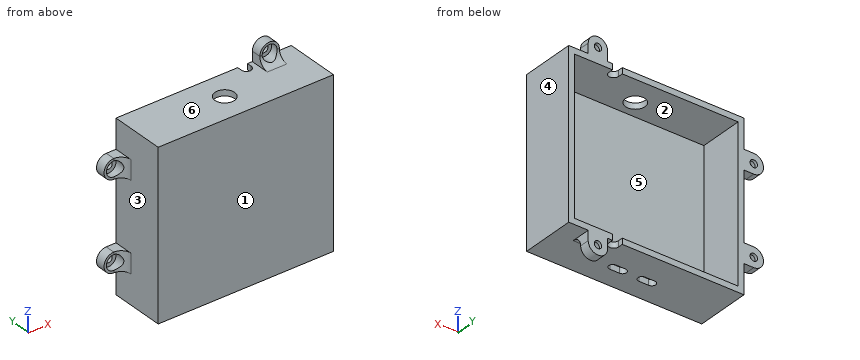
from build123d import *

# Parameters (mm, degrees)
SKETCH1_W                                      = 90
SKETCH1_H                                      = 85
BOSS_EXTRUDE1_DEPTH                            = 28
SHELL1_T                                       = -3
SHELL1_THICKNESS_2_FACE_W                      = 79
SHELL1_THICKNESS_2_FACE_H                      = 84
SHELL1_THICKNESS_2_DEPTH                       = 2.25
CUT_EXTRUDE1_REACH                             = 102.17
SKETCH2_R                                      = 5.05
BOSS_EXTRUDE2_DEPTH                            = 5
BOSS_EXTRUDE3_DEPTH                            = 5
CBORE_FOR_6_SOCKET_HEAD_CAP_SCREW1_D           = 3.7973
CBORE_FOR_6_SOCKET_HEAD_CAP_SCREW1_CBORE_D     = 7.62
CBORE_FOR_6_SOCKET_HEAD_CAP_SCREW1_CBORE_DEPTH = 3.5052
FILLET1_R                                      = 5
CUT_EXTRUDE2_DEPTH                             = 114.287245531
CUT_EXTRUDE4_REACH                             = 124.741


with BuildPart() as part:
    # Sketch1 → Boss-Extrude1 (new body)
    with BuildSketch(Plane(origin=(0, 0, 0), x_dir=(1, 0, 0), z_dir=(0, 1, 0))):
        Rectangle(SKETCH1_W, SKETCH1_H)
    extrude(amount=BOSS_EXTRUDE1_DEPTH)

    # Shell1
    shell1_openings = [part.faces().sort_by_distance(p)[0] for p in [
        (0, 28, 0),
    ]]
    offset(amount=SHELL1_T, openings=shell1_openings, kind=Kind.INTERSECTION)

    # Shell1 thickness 2 face (on inner face of the shell) → Shell1 thickness 2 (add)
    with BuildSketch(Plane(origin=(0, 3, 0), x_dir=(0, 0, -1), z_dir=(0, -1, 0))):
        Rectangle(SHELL1_THICKNESS_2_FACE_W, SHELL1_THICKNESS_2_FACE_H)
    extrude(amount=-SHELL1_THICKNESS_2_DEPTH)

    # Sketch2 → Cut-Extrude1 (cut, up to next)
    with BuildSketch(Plane.XY.offset(42.5), mode=Mode.PRIVATE) as cut_extrude1_sk1:
        with Locations((0, 14)):
            Circle(SKETCH2_R)
    cut_extrude1_tool1 = extrude(cut_extrude1_sk1.sketch, amount=-CUT_EXTRUDE1_REACH, mode=Mode.PRIVATE) & part.part
    add(cut_extrude1_tool1.solids().sort_by_distance((0, 14, 42.5))[0], mode=Mode.SUBTRACT)

    # Sketch3 → Boss-Extrude2 (add)
    with BuildSketch(Plane(origin=(0, 28, 0), x_dir=(1, 0, 0), z_dir=(0, 1, 0))):
        with BuildLine():
            Line((-50, 27.5), (-45, 27.5))
            Line((-45, 27.5), (-45, 17.5))
            Line((-45, 17.5), (-50, 17.5))
            ThreePointArc((-50, 17.5), (-55, 22.5), (-50, 27.5))
        make_face()
    boss_extrude2 = extrude(amount=-BOSS_EXTRUDE2_DEPTH)

    # Mirror1: Boss-Extrude2 across plane
    add(boss_extrude2.mirror(Plane.XY))

    # Sketch4 → Boss-Extrude3 (add)
    with BuildSketch(Plane(origin=(0, 28, 0), x_dir=(1, 0, 0), z_dir=(0, 1, 0))):
        with BuildLine():
            Line((25, 47.5), (25, 42.5))
            Line((25, 42.5), (35, 42.5))
            Line((35, 42.5), (35, 47.5))
            ThreePointArc((35, 47.5), (30, 52.5), (25, 47.5))
        make_face()
    boss_extrude3 = extrude(amount=-BOSS_EXTRUDE3_DEPTH)

    # Mirror2: Boss-Extrude3 across plane
    add(boss_extrude3.mirror(Plane.XY))

    # CBORE for #6 Socket Head Cap Screw1 (through all)
    with Locations(Plane(origin=(0, 23, 0), x_dir=(-1, 0, 0), z_dir=(0, -1, 0))):
        with Locations((-30, 47.5), (-30, -47.5), (50, -22.5), (50, 22.5)):
            CounterBoreHole(CBORE_FOR_6_SOCKET_HEAD_CAP_SCREW1_D / 2, CBORE_FOR_6_SOCKET_HEAD_CAP_SCREW1_CBORE_D / 2, CBORE_FOR_6_SOCKET_HEAD_CAP_SCREW1_CBORE_DEPTH)

    # Fillet1
    # the kernel refuses this fillet: 5 mm, written as the material it adds along each edge
    with BuildSketch(Plane(origin=(25, 23, -42.5), x_dir=(0, -1, 0), z_dir=(1, 0, 0))) as fillet1_piece_1_section:
        with BuildLine():
            CenterArc((FILLET1_R, FILLET1_R), FILLET1_R, 180, 90)
            Line((0, FILLET1_R), (0, 0))
            Line((0, 0), (FILLET1_R, 0))
        make_face()
    fillet1_piece_1 = extrude(amount=10, mode=Mode.PRIVATE)
    fillet1_piece_1 = fillet1_piece_1 - Plane(origin=(30, 21.803509944, -47.5), x_dir=(-1, 0, 0), z_dir=(0, -1, 0)) * Cylinder(3.81, 40, mode=Mode.PRIVATE)
    add(fillet1_piece_1)
    with BuildSketch(Plane(origin=(25, 23, 42.5), x_dir=(0, -1, 0), z_dir=(1, 0, 0))) as fillet1_piece_2_section:
        with BuildLine():
            CenterArc((FILLET1_R, -FILLET1_R), FILLET1_R, 90, 90)
            Line((0, -FILLET1_R), (0, 0))
            Line((0, 0), (FILLET1_R, 0))
        make_face()
    fillet1_piece_2 = extrude(amount=10, mode=Mode.PRIVATE)
    fillet1_piece_2 = fillet1_piece_2 - Plane(origin=(30, 21.803509344, 47.5), x_dir=(-1, 0, 0), z_dir=(0, -1, 0)) * Cylinder(3.81, 40, mode=Mode.PRIVATE)
    add(fillet1_piece_2)
    with BuildSketch(Plane(origin=(-45, 23, -27.5), x_dir=(0, -1, 0), z_dir=(0, 0, 1))) as fillet1_piece_3_section:
        with BuildLine():
            CenterArc((FILLET1_R, -FILLET1_R), FILLET1_R, 90, 90)
            Line((0, -FILLET1_R), (0, 0))
            Line((0, 0), (FILLET1_R, 0))
        make_face()
    fillet1_piece_3 = extrude(amount=10, mode=Mode.PRIVATE)
    fillet1_piece_3 = fillet1_piece_3 - Plane(origin=(-50, 21.803509344, -22.5), x_dir=(-1, 0, 0), z_dir=(0, -1, 0)) * Cylinder(3.81, 40, mode=Mode.PRIVATE)
    add(fillet1_piece_3)
    with BuildSketch(Plane(origin=(-45, 23, 27.5), x_dir=(0, -1, 0), z_dir=(0, 0, -1))) as fillet1_piece_4_section:
        with BuildLine():
            CenterArc((FILLET1_R, FILLET1_R), FILLET1_R, 180, 90)
            Line((0, FILLET1_R), (0, 0))
            Line((0, 0), (FILLET1_R, 0))
        make_face()
    fillet1_piece_4 = extrude(amount=10, mode=Mode.PRIVATE)
    fillet1_piece_4 = fillet1_piece_4 - Plane(origin=(-50, 21.803509944, 22.5), x_dir=(-1, 0, 0), z_dir=(0, -1, 0)) * Cylinder(3.81, 40, mode=Mode.PRIVATE)
    add(fillet1_piece_4)

    # Sketch9 → Cut-Extrude2 (cut, through all)
    with BuildSketch(Plane.XY.offset(42.5)):
        with BuildLine():
            Line((22.5, 28), (22.5, 25.5))
            ThreePointArc((22.5, 25.5), (20, 23), (17.5, 25.5))
            Line((17.5, 25.5), (17.5, 28))
            ThreePointArc((17.5, 28), (20, 30.5), (22.5, 28))
        make_face()
    extrude(amount=-CUT_EXTRUDE2_DEPTH, mode=Mode.SUBTRACT)

    # Sketch10 → Cut-Extrude4 (cut, up to next)
    with BuildSketch(Plane(origin=(17.5, 0, -42.5), x_dir=(1, 0, 0), z_dir=(0, 0, 1)), mode=Mode.PRIVATE) as cut_extrude4_sk1:
        with BuildLine():
            Line((-27.5, 14), (-22.5, 14))
            ThreePointArc((-22.5, 14), (-20.5, 12), (-22.5, 10))
            Line((-22.5, 10), (-27.5, 10))
            ThreePointArc((-27.5, 10), (-29.5, 12), (-27.5, 14))
        make_face()
    cut_extrude4_tool1 = extrude(cut_extrude4_sk1.sketch, amount=CUT_EXTRUDE4_REACH, mode=Mode.PRIVATE) & part.part
    # Sketch10 → Cut-Extrude4 (cut, up to next)
    with BuildSketch(Plane(origin=(17.5, 0, -42.5), x_dir=(1, 0, 0), z_dir=(0, 0, 1)), mode=Mode.PRIVATE) as cut_extrude4_sk2:
        with BuildLine():
            Line((-7.5, 14), (-12.5, 14))
            ThreePointArc((-12.5, 14), (-14.5, 12), (-12.5, 10))
            Line((-12.5, 10), (-7.5, 10))
            ThreePointArc((-7.5, 10), (-5.5, 12), (-7.5, 14))
        make_face()
    cut_extrude4_tool2 = extrude(cut_extrude4_sk2.sketch, amount=CUT_EXTRUDE4_REACH, mode=Mode.PRIVATE) & part.part
    add(cut_extrude4_tool1.solids().sort_by_distance((-7.5, 12, -42.5))[0], mode=Mode.SUBTRACT)
    add(cut_extrude4_tool2.solids().sort_by_distance((7.5, 12, -42.5))[0], mode=Mode.SUBTRACT)


solid = part.part
The model under review builds one solid part; all positions refer to its coordinate system, in mm. Face numbers are marked on the shaded views. A direction names the side the tool comes from. Coordinates: 2 decimals unless noted, no trailing zeros. Loops run counter-clockwise (first coordinate to the right, second up) from the corner with the lowest first, then second, coordinate; pieces in that order, holes last. Notation, with made-up numbers: M -25,21 L -10,21 A29 cw -10,46 Z; hole C 81.5,25 d1. An arc over 180 degrees is marked long. Put each result on its own line as item: value. Start each with the question number.
Q1. The part is to be moulded in two halves that separate along X. For the marked faces 4, 5 and 6, say which applies: +X half, -X half, draft (parallel to the pull), parting line (faces both ways), or undercut.
Q2. Wall thickness on line 1 (Z direction, x = -50, y = 24); line 2 (X direction, y = 24.55, z = 22.5); line 3 (Z direction, x = 30, y = 27.1): over which ranges is each line inside the solid? List them lowest first.
Q3. Add section A-A (z = 22.5). Write out the cut boundary in (x, y).
Q4. For the marked faces 1, 2 and 3, list the 3-axis set-ups (+Z, -Z, +X, -X, +Y, -Y) from which the entire face can be reached by the end or side of a thin tool; tool diameter is ignored.
Q5. Add section B-B (x = 30). Write out the cut boundary in (y, z).
Q6. Add section C-C (y = 12). Write out the cut boundary in (x, z).
Q7. Add section D-D (x = -19.5). Write out the cut boundary in (y, z).
Q8. Clearance check with flat-ended pins moving along their axes: pin 1 (2.5 mm diameter, centred on y = 25, z = -45, fed in from +X); pin 2 (2 mm diameter, centred on y = 26.5, z = -41, fed in from -X); pin 3 (12 mm diameter, centred on x = -15, y = 11.5, fed in from +Z). State where each tip first meets the part, or that it passes through.
Answers:
1. face 4: +X half
1. face 5: undercut
1. face 6: draft
2. line 1: z = -27.5 to -26.31, -18.69 to -17.5, 17.5 to 18.69, 26.31 to 27.5
2. line 2: x = -55 to -53.81, -46.19 to -42, 42 to 45
2. line 3: z = -52.5 to -49.4, -45.6 to -39.5, 39.5 to 45.6, 49.4 to 52.5
3. outline: M -55,23 L -53.81,23 L -53.81,26.51 L -51.9,26.51 L -51.9,28 L -55,28 Z; M -48.1,26.51 L -46.19,26.51 L -46.19,21.24 A5 cw -45,18 L -45,0 L 45,0 L 45,28 L 42,28 L 42,5.25 L -42,5.25 L -42,28 L -48.1,28 Z
4. face 1: +Z, -Z, +X, -X, -Y
4. face 2: +Y
4. face 3: -X, -Y
5. outline: M 0,-42.5 L 18,-42.5 A5 cw 21.24,-43.69 L 26.51,-43.69 L 26.51,-45.6 L 28,-45.6 L 28,-39.5 L 5.25,-39.5 L 5.25,39.5 L 28,39.5 L 28,45.6 L 26.51,45.6 L 26.51,43.69 L 21.24,43.69 A5 cw 18,42.5 L 0,42.5 Z; M 23,-52.5 L 28,-52.5 L 28,-49.4 L 26.51,-49.4 L 26.51,-51.31 L 23,-51.31 Z; M 23,51.31 L 26.51,51.31 L 26.51,49.4 L 28,49.4 L 28,52.5 L 23,52.5 Z
6. outline: M -45,-42.5 L -12,-42.5 L -12,-39.5 L -42,-39.5 L -42,39.5 L -4.64,39.5 L -4.64,42.5 L -45,42.5 Z; M -3,-42.5 L 3,-42.5 L 3,-39.5 L -3,-39.5 Z; M 4.64,39.5 L 42,39.5 L 42,-39.5 L 12,-39.5 L 12,-42.5 L 45,-42.5 L 45,42.5 L 4.64,42.5 Z
7. outline: M 0,-42.5 L 28,-42.5 L 28,-39.5 L 5.25,-39.5 L 5.25,39.5 L 28,39.5 L 28,42.5 L 0,42.5 Z
8. pin 1: stops at x = 35
8. pin 2: stops at x = -45
8. pin 3: stops at z = 42.5
